```python
from build123d import *

# Parameters (mm, degrees)
F0_W      = 177.8
F0_H      = 47.6504
F1_DEPTH  = 76.2
F2_R      = 4.7752
F2_R_2    = 1.9812
F3_DEPTH  = 47.6514
F5_DEPTH  = 16.002
F7_DEPTH  = 33.528
F9_DEPTH  = 31.7246
F11_DEPTH = 31.7246


with BuildPart() as f1:
    # F0 (on Top) → F1 (new body)
    with BuildSketch(Plane.XY):
        with Locations((88.911714, 52.4002)):
            Rectangle(F0_W, F0_H)
    extrude(amount=F1_DEPTH)

    # F2 (on face) → F3 (cut, through all)
    with BuildSketch(Plane.XZ.offset(-28.575)):
        with Locations((146.303014, 58.0644)):
            Circle(F2_R)
        with Locations((117.728014, 52.3494)):
            Circle(F2_R_2)
        with Locations((96.315814, 60.325)):
            Circle(F2_R_2)
    extrude(amount=-F3_DEPTH, mode=Mode.SUBTRACT)

    # F4 (on face) → F5 (cut)
    with BuildSketch(Plane.XY.offset(76.2)):
        with BuildLine():
            Line((176.910014, 51.587385), (176.910014, 53.214231))
            ThreePointArc((176.910014, 53.214231), (175.329273, 57.08812), (171.489579, 58.7502))
            Line((171.489579, 58.7502), (151.347379, 58.7502))
            ThreePointArc((151.347379, 58.7502), (145.959225, 56.518354), (143.727379, 51.1302))
            Line((143.727379, 51.1302), (143.727379, 49.2252))
            ThreePointArc((143.727379, 49.2252), (144.657315, 46.980136), (146.902379, 46.0502))
            Line((146.902379, 46.0502), (171.385514, 46.0502))
            ThreePointArc((171.385514, 46.0502), (175.292693, 47.676486), (176.910014, 51.587385))
        make_face()
    extrude(amount=-F5_DEPTH, mode=Mode.SUBTRACT)

    # F6 (on face) → F7 (cut)
    with BuildSketch(Plane.XY.offset(76.2)):
        with BuildLine():
            Line((117.829614, 56.3626), (108.482414, 56.3626))
            ThreePointArc((108.482414, 56.3626), (105.680574, 55.20204), (104.520014, 52.4002))
            ThreePointArc((104.520014, 52.4002), (105.680574, 49.59836), (108.482414, 48.4378))
            Line((108.482414, 48.4378), (117.829614, 48.4378))
            ThreePointArc((117.829614, 48.4378), (120.631454, 49.59836), (121.792014, 52.4002))
            ThreePointArc((121.792014, 52.4002), (120.631454, 55.20204), (117.829614, 56.3626))
        make_face()
    extrude(amount=-F7_DEPTH, mode=Mode.SUBTRACT)

    # F8 (on face) → F9 (cut)
    with BuildSketch(Plane.XY.offset(76.2)):
        with BuildLine():
            Line((134.771414, 61.1632), (93.242414, 61.1632))
            ThreePointArc((93.242414, 61.1632), (89.327022, 59.541392), (87.705214, 55.626))
            Line((87.705214, 55.626), (87.705214, 49.1744))
            ThreePointArc((87.705214, 49.1744), (89.327022, 45.259008), (93.242414, 43.6372))
            Line((93.242414, 43.6372), (134.771414, 43.6372))
            ThreePointArc((134.771414, 43.6372), (138.686805, 45.259008), (140.308614, 49.1744))
            Line((140.308614, 49.1744), (140.308614, 55.626))
            ThreePointArc((140.308614, 55.626), (138.686805, 59.541392), (134.771414, 61.1632))
        make_face()
    extrude(amount=-F9_DEPTH, mode=Mode.SUBTRACT)

    # F10 (on face) → F11 (cut)
    with BuildSketch(Plane.XY.offset(76.2)):
        with BuildLine():
            Line((147.242814, 57.1754), (139.34862, 57.1754))
            ThreePointArc((139.34862, 57.1754), (137.103556, 56.245464), (136.17362, 54.0004))
            Line((136.17362, 54.0004), (136.17362, 49.2252))
            ThreePointArc((136.17362, 49.2252), (137.103556, 46.980136), (139.34862, 46.0502))
            Line((139.34862, 46.0502), (147.242814, 46.0502))
            ThreePointArc((147.242814, 46.0502), (151.158205, 47.672008), (152.780014, 51.5874))
            Line((152.780014, 51.5874), (152.780014, 51.6382))
            ThreePointArc((152.780014, 51.6382), (151.158205, 55.553592), (147.242814, 57.1754))
        make_face()
    extrude(amount=-F11_DEPTH, mode=Mode.SUBTRACT)


solid = f1.part
```
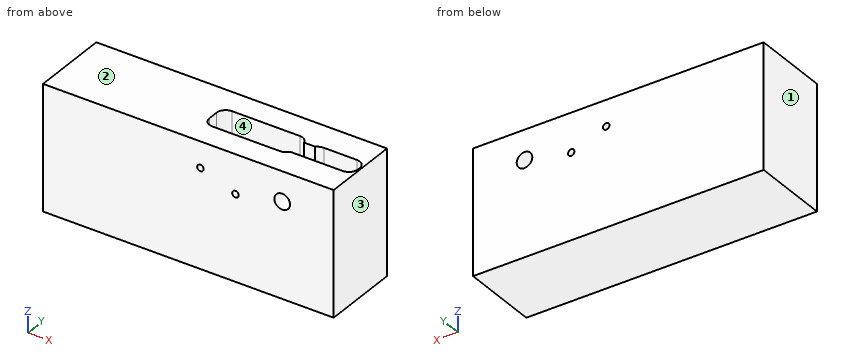
Input: part model. Units: mm. Frame: model coordinates. Face numbers are marked on the shaded views. Round coordinates to 2 decimals unless told otherwise and drop trailing zeros. Loops run counter-clockwise (first coordinate to the right, second up) from the corner with the lowest first, then second, coordinate; pieces in that order, holes last. Notation, with made-up numbers: (31.5, 61) -> (81.5, 61) arc R12 ccw to (81.5, 69) -> close; hole circle Ø4 at (64, -10.75). An arc over 180 degrees is marked (long way). One line per item, written item: value.
(1) Section B-B (x = 102). Return the cut outline in (y, z) (3 decimals), plus the area to 3 significant figures.
Geometry check:
outline: (28.575, 0) -> (76.225, 0) -> (76.225, 76.2) -> (61.163, 76.2) -> (61.163, 44.475) -> (43.637, 44.475) -> (43.637, 76.2) -> (28.575, 76.2) -> close
area: 3,070 mm2
(2) Material intervals for line 1 (Y direction, x = 117, z = 69) (3 decimals); line 2 (X direction, y = 35.5, z = 54); line 3 (X direction, y = 74.5, z = 51.5), sorted ascending. Write a range as [from, to].
Geometry check:
line 1: [28.575, 43.637], [61.163, 76.225]
line 2: [0.01, 116.63], [118.82, 143.8], [148.81, 177.81]
line 3: [0.01, 115.94], [119.52, 177.81]
(3) Mould query, pull axis X, two halves, no side actions, for the marked faces 1, 2, 3 and 4. Classes: pulls with the +X half, pulls with the -X half, needs draft (parallel to the pull), parting line crosses it, or undercut.
Geometry check:
face 1: pulls with the -X half
face 2: needs draft
face 3: pulls with the +X half
face 4: undercut
(4) Pin query (flat end, axial travel): pin 1 (5 mm diameter, centred on x = 117.73, z = 52.35, fed in from +Y); pin 2 (2.5 mm diameter, centred on x = 113.5, y = 51.5, fed in from +Z). Return the tip coordinate at first contact, or that it passes through.
Geometry check:
pin 1: y = 76.23
pin 2: z = 42.67
(5) Section A-A (z = 56). Return the cut outline in (x, y) (3 decimals), plus the area to 3 significant figures.
Geometry check:
outline: (0.012, 28.575) -> (141.997, 28.575) -> (141.997, 46.05) -> (139.349, 46.05) arc R3.175 cw to (139.343, 46.05) arc R5.537 cw to (134.771, 43.637) -> (93.242, 43.637) arc R5.537 cw to (87.705, 49.174) -> (87.705, 55.626) arc R5.537 cw to (93.242, 61.163) -> (134.771, 61.163) arc R5.537 cw to (140.087, 57.175) -> (141.997, 57.175) -> (141.997, 76.225) -> (0.012, 76.225) -> close; (150.609, 28.575) -> (177.812, 28.575) -> (177.812, 76.225) -> (150.609, 76.225) -> (150.609, 56.035) arc R5.537 cw to (152.78, 51.638) -> (152.78, 51.587) arc R5.537 cw to (150.609, 47.191) -> close
area: 7,130 mm2
